Part model, mm, in its own coordinate system. A direction names the side the tool comes from. Give positions to 0.01 mm unless a question says otherwise; leave off trailing zeros. Order: outer loops, then holes, each group sorted by start corner. A loop starts at its lowest first (then second) coordinate and runs counter-clockwise, first axis right, second up. Notation, with made-up numbers: M 33.25,-19 L 76.25,-19 A24 cw 76.25,9 Z; hole C 4.25,4 d8. An arc over 180 degrees is marked long. Answer as a JSON object with one key per item and string values.
from build123d import *

# Parameters (mm, degrees)
SKETCH1_W               = 160
SKETCH1_H               = 70
BOSS_EXTRUDE1_DEPTH     = 7.5
CUT_EXTRUDE1_DEPTH      = 88.642740715
CUT_EXTRUDE1_DEPTH_BACK = 88.642740715
SKETCH2_R               = 2.5
SKETCH2_R_2             = 3
SKETCH3_R               = 4.5
CUT_EXTRUDE2_DEPTH      = 5.5
SKETCH4_R               = 5
CUT_EXTRUDE3_DEPTH      = 6
SKETCH5_W               = 95
SKETCH5_H               = 5
BOSS_EXTRUDE2_DEPTH     = 2.3
BOSS_EXTRUDE3_DEPTH     = 95
FILLET1_R               = 1
FILLET2_R               = 0.5
FILLET3_R               = 10


with BuildPart() as part:
    # Sketch1 → Boss-Extrude1 (new body)
    with BuildSketch(Plane.XY):
        Rectangle(SKETCH1_W, SKETCH1_H)
    extrude(amount=BOSS_EXTRUDE1_DEPTH)

    # Sketch2 → Cut-Extrude1 (cut, two sides: drawn at the far end of the back side and taken through both)
    with BuildSketch(Plane.XY.offset(7.5).offset(-CUT_EXTRUDE1_DEPTH_BACK)):
        with Locations((-70, 0)):
            Circle(SKETCH2_R)
        with Locations((60, 0)):
            Circle(SKETCH2_R_2)
    extrude(amount=CUT_EXTRUDE1_DEPTH + CUT_EXTRUDE1_DEPTH_BACK, mode=Mode.SUBTRACT)

    # Sketch3 → Cut-Extrude2 (cut)
    with BuildSketch(Plane.XY.offset(7.5)):
        with Locations((-70, 0)):
            Circle(SKETCH3_R)
    extrude(amount=-CUT_EXTRUDE2_DEPTH, mode=Mode.SUBTRACT)

    # Sketch4 → Cut-Extrude3 (cut)
    with BuildSketch(Plane(origin=(0, 0, 0), x_dir=(-1, 0, 0), z_dir=(0, 0, -1))):
        with Locations((-60, 0)):
            Circle(SKETCH4_R)
    extrude(amount=-CUT_EXTRUDE3_DEPTH, mode=Mode.SUBTRACT)

    # Sketch5 → Boss-Extrude2 (add)
    with BuildSketch(Plane(origin=(0, 0, 0), x_dir=(-1, 0, 0), z_dir=(0, 0, -1))):
        with Locations((12.5, 0)):
            Rectangle(SKETCH5_W, SKETCH5_H)
    extrude(amount=BOSS_EXTRUDE2_DEPTH)

    # Sketch6 → Boss-Extrude3 (add)
    with BuildSketch(Plane(origin=(35, 0, 0), x_dir=(0, 0, -1), z_dir=(1, 0, 0))):
        Polygon((2.3, 6), (2.3, -6), (6.6, -2.5), (6.6, 2.5), align=None)
    extrude(amount=-BOSS_EXTRUDE3_DEPTH)

    # Fillet1
    fillet1_edges = [part.edges().sort_by_distance(p)[0] for p in [
        (-12.5, -2.5, -6.6),
        (-12.5, 2.5, -6.6),
    ]]
    fillet(fillet1_edges, radius=FILLET1_R)

    # Fillet2
    fillet2_edges = [part.edges().sort_by_distance(p)[0] for p in [
        (-12.5, -6, -2.3),
        (-12.5, 6, -2.3),
    ]]
    fillet(fillet2_edges, radius=FILLET2_R)

    # Fillet3
    fillet3_edges = [part.edges().sort_by_distance(p)[0] for p in [
        (-80, 35, 3.75),
        (80, 35, 3.75),
        (80, -35, 3.75),
        (-80, -35, 3.75),
    ]]
    fillet(fillet3_edges, radius=FILLET3_R)


solid = part.part
1. Probe line 1 along Y through (x, z) = (-70, 6.1); line 2 along Y through (x, z) = (60, 6.55); line 3 along Z through (x, y) = (52.5, 30). List the from-to ranges inside material, lowest first.
Worked answers:
{"line 1": "y = -35 to -4.5, 4.5 to 35", "line 2": "y = -35 to -3, 3 to 35", "line 3": "z = 0 to 7.5"}
2. Cut at A-A on x = 60. Give the cut face in (y, z).
Worked answers:
{"outline": "M -35,0 L -5,0 L -5,6 L -3,6 L -3,7.5 L -35,7.5 Z; M 3,6 L 5,6 L 5,0 L 35,0 L 35,7.5 L 3,7.5 Z"}
3. Cut at C-C on x = 7. Give the cut face in (y, z), plus the area to 4 significant figures.
Worked answers:
{"outline": "M -35,0 L -2.5,0 L -2.5,-2.3 L -4.95,-2.3 A0.5 ccw -5.34,-3.12 L -2.8,-6.23 A1 ccw -2.02,-6.6 L 2.02,-6.6 A1 ccw 2.8,-6.23 L 5.34,-3.12 A0.5 ccw 4.95,-2.3 L 2.5,-2.3 L 2.5,0 L 35,0 L 35,7.5 L -35,7.5 Z", "area": "572.5 mm^2"}
4. Which spindle directions (+Z, -Z, +X, -X, +Y, -Y) get a long thin tool onto all of the face, cutting with end or side? Do faces 5 (the flat face through (35, 0, -3)), 6 (the flat face through (-68, -2, 2)), 7 (the flat face through (-60, 0, -3)). Say none if no direction does.
Worked answers:
{"face 5": "-Z, +X, +Y, -Y", "face 6": "+Z", "face 7": "-Z, -X, +Y, -Y"}
5. Two-plate mould, pull along Y, no slides. Class faces 1 (the cylindrical face through (57, 0, 7)), 2 (the cylindrical face through (-72, -1.5, 1)), 3 (the flat face through (80, 0, 4)), 4 (the cylindrical face through (-77.15, 31.99, 3.8)): +Y half, -Y half, draft (parallel to the pull), parting line (faces both ways), or undercut.
Worked answers:
{"face 1": "undercut", "face 2": "undercut", "face 3": "draft", "face 4": "+Y half"}
6. Cut at D-D on y = -9. Give the cut face in (x, z).
Worked answers:
{"outline": "M -80,0 L 80,0 L 80,7.5 L -80,7.5 Z"}
7. Pin check, flat tips, straight feed: P1, Ø3, axis at x = -32, z = -4.5, coming from the +Y side; P2, Ø4, axis at x = -70, y = 0, coming from the +Z side; P3, Ø2, axis at x = 16, y = 11.5, coming from the -Z side; P4, Ø0.7, axis at x = -13, z = -1, coming from the -Y side. Stop position of each tip, or through.
Worked answers:
{"P1": "stops at y = 5.41", "P2": "passes through", "P3": "stops at z = 0", "P4": "stops at y = -2.5"}
8. Cut at B-B on z = 3.5. Give the cut face in (x, y).
Worked answers:
{"outline": "M -80,-25 A10 ccw -70,-35 L 70,-35 A10 ccw 80,-25 L 80,25 A10 ccw 70,35 L -70,35 A10 ccw -80,25 Z; hole C -70,0 d9; hole C 60,0 d10"}
